from build123d import *

# Parameters (mm, degrees)
F0_W     = 127
F0_H     = 127
F1_DEPTH = 127
F4_DEPTH = 101.6
F5_R     = 6.35
F6_DEPTH = 203.2
F7_T     = -2.54


with BuildPart() as f1:
    # F0 (on Front) → F1 (new body)
    with BuildSketch(Plane.XZ):
        with Locations((-1.222377643, -1.6671840248)):
            Rectangle(F0_W, F0_H)
    extrude(amount=F1_DEPTH)

    # F3 (on face) + F2 (on face) → F4 (cut)
    with BuildSketch(Plane.XY.offset(61.8328159752)):
        Polygon((62.8832024596, -127.1058379948), (62.8832024596, -76.3058379948), (12.0832024596, -127.1058379948), align=None)
    with BuildSketch(Plane.XY.offset(61.8328159752)):
        Polygon((-13.922377643, 0), (-64.722377643, 0), (-64.722377643, -50.8), align=None)
    extrude(amount=-F4_DEPTH, mode=Mode.SUBTRACT)

    # F5 (on face) → F6 (cut)
    with BuildSketch(Plane.XY.offset(-39.7671840248)):
        with Locations((-49.482377643, -15.24)):
            Circle(F5_R)
        with Locations((47.037622357, -111.76)):
            Circle(F5_R)
    extrude(amount=-F6_DEPTH, mode=Mode.SUBTRACT)

    # F7
    f7_openings = [f1.faces().sort_by_distance(p)[0] for p in [
        (-1.222378, -63.5, -65.167184),
    ]]
    offset(amount=F7_T, openings=f7_openings, kind=Kind.INTERSECTION)


solid = f1.part
Check sheet for the modelled part. Datum: model origin and axes. Units: mm. A direction names the side the tool comes from. Give positions to 0.01 mm unless a question says otherwise; leave off trailing zeros. Loops run counter-clockwise (first coordinate to the right, second up) from the corner with the lowest first, then second, coordinate; pieces in that order, holes last. Notation, with made-up numbers: M 43.5,34 L 86.5,34 A10 ccw 86.5,46 Z; hole C 89,-36.5 d7. An arc over 180 degrees is marked long. Use a Markdown table: item, result. Add a question column.
Q1. Sectioned sample at B-B, the plane x = 45. Record the cut outline in (y, z).
Q2. Tool access check on faces 1 (the flat face through (-2, -63, 61.833)), 2 (the flat face through (-39.68, -25.76, 11.74)), 3 (the flat face through (42, -107, -39.767)), 4 (the flat face through (41, -105, -42.307)). Record the directions out of +Z, -Z, +X, -X, +Y, -Y that give a thin tool (end or side, any length) a straight path to the whole face; none if there is none.
Q3. Mould release check, pull along X, two halves, no side actions. Record for faces 5 (the flat face through (-38, -21, -42.307)), 6 (the flat face through (62.278, -48, -3)), 7 (the cylindrical face through (45.88, -102.946, -53.577)), 8 (the flat face through (-16, -127, -1)): pulls with the +X half, pulls with the -X half, needs draft (parallel to the pull), parting line crosses it, or undercut.
Q4. Sectioned sample at D-D, the plane x = 32. Record the cut outline in (y, z), then the cut area to 3 significant figures.
Q5. Sectioned sample at C-C, the plane y = -111.76. Record the cut outline in (x, z).
Q6. Scan lines: line 1 along X through (y, z) = (-15, -59); line 2 along Y through (x, z) = (17, -52.5); line 3 along X through (y, z) = (-70, 24). Record each from-to range of solid material in increasing order. Write a range as [from, to].
Q7. Sectioned sample at A-A, the plane z = 19. Record the cut outline in (x, y), then the cut area to 3 significant figures.
Q8. Go/stop test with flat-tipped pins: pin 1 (1.5 mm diameter, centred on x = -20, z = 48, fed in from +Y); pin 2 (12 mm diameter, centred on x = 23.5, y = -72.5, fed in from -Z); pin 3 (1 mm diameter, centred on x = -26, z = 33, fed in from +Y). Record where each tip stops, or that it passes through.
Verdict:
| question | item | result |
|---|---|---|
| 1 | outline | M -127,-65.17 L -124.46,-65.17 L -124.46,-42.31 L -120.41,-42.31 L -120.41,-65.17 L -117.77,-65.17 L -117.77,-39.77 L -127,-39.77 Z; M -105.75,-65.17 L -103.11,-65.17 L -103.11,-42.31 L -90.6,-42.31 L -90.6,59.29 L -2.54,59.29 L -2.54,-65.17 L 0,-65.17 L 0,61.83 L -94.19,61.83 L -94.19,-39.77 L -105.75,-39.77 Z |
| 2 | face 1 | +Z, +X, -X, +Y, -Y |
| 2 | face 2 | +Z, -X, +Y |
| 2 | face 3 | +Z, +X, -Y |
| 2 | face 4 | -Z |
| 3 | face 5 | undercut |
| 3 | face 6 | pulls with the +X half |
| 3 | face 7 | undercut |
| 3 | face 8 | needs draft |
| 4 | outline | M -127,-65.17 L -124.46,-65.17 L -124.46,-42.31 L -103.6,-42.31 L -103.6,59.29 L -2.54,59.29 L -2.54,-65.17 L 0,-65.17 L 0,61.83 L -107.19,61.83 L -107.19,-39.77 L -127,-39.77 Z |
| 4 | area | 1,060 mm^2 |
| 5 | outline | M -64.72,-65.17 L -62.18,-65.17 L -62.18,59.29 L 23.84,59.29 L 23.84,-42.31 L 38.15,-42.31 L 38.15,-65.17 L 40.69,-65.17 L 40.69,-39.77 L 27.43,-39.77 L 27.43,61.83 L -64.72,61.83 Z; M 53.39,-65.17 L 55.93,-65.17 L 55.93,-42.31 L 59.74,-42.31 L 59.74,-65.17 L 62.28,-65.17 L 62.28,-39.77 L 53.39,-39.77 Z |
| 6 | line 1 | [-64.72, -62.18], [-58.37, -55.83], [-43.14, -40.6], [59.74, 62.28] |
| 6 | line 2 | [-127, -124.46], [-2.54, 0] |
| 6 | line 3 | [-64.72, -62.18], [59.74, 62.28] |
| 7 | outline | M -64.72,-127 L 12.19,-127 L 62.28,-76.91 L 62.28,0 L -13.92,0 L -64.72,-50.8 Z; hole M -62.18,-124.46 L 11.14,-124.46 L 59.74,-75.86 L 59.74,-2.54 L -12.87,-2.54 L -62.18,-51.85 Z |
| 7 | area | 1,120 mm^2 |
| 8 | pin 1 | y = -5.33 |
| 8 | pin 2 | z = 59.29 |
| 8 | pin 3 | y = -11.58 |
